Autodesk Inventor part; units mm, degrees
ref_plane "YZ Plane" through (0, 0, 0) normal (1, 0, 0) x (0, 1, 0)
ref_plane "XZ Plane" through (0, 0, 0) normal (0, 1, 0) x (-1, 0, 0)
ref_plane "XY Plane" through (0, 0, 0) normal (0, 0, 1) x (1, 0, 0)
sketch "スケッチ2" plane through (0, 0, 0) normal (1, 0, 0) x (0, 1, 0)
  line L0 (-7.071, 15.2913) -> (-10.3324, 22.2065)
  arc A0 (-10.3324, 22.2065) -> (0.9209, 24.5984) centre (0.1387, 0.6112) ccw
  line L1 (0.9209, 24.5984) -> (0.7542, 16.9546)
  line L2 (0.7542, 16.9546) -> (-7.071, 15.2913)
  circle A1 centre (-8.8613, 0.6112) radius 1.6
  circle A2 centre (9.1387, 0.6112) radius 1.6
  circle A3 centre (0.1387, 0.6112) radius 5.15
  point P0 (0, 0)
extrude "押し出し2" add sketch "スケッチ2" along normal blind 2.5
properties part number "belt_liner_v2_3DP_P-4-F" material "ABS プラスチック"
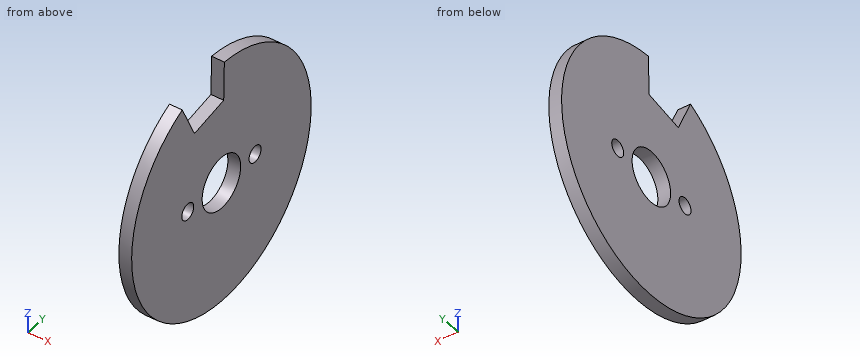
Part model, mm, in its own coordinate system. Round coordinates to 2 decimals unless told otherwise and drop trailing zeros. Write each loop counter-clockwise with the first axis right and the second up, starting at its lowest first coordinate (ties: lowest second). Pieces come first, ordered by that corner, then holes. Notation, with made-up numbers: M 55,87 L 103,87 A16 cw 103,117 Z; hole C 56.5,84 d5. An arc over 180 degrees is marked long. One line per question, with ' | ' between items.
(1) Probe line 1 along Z through (x, y) = (1.75, -3.5); line 2 along Y through (x, z) = (1.85, -4); line 3 along Z through (x, y) = (1.85, 2.5). List the from-to ranges inside material, lowest first.
Answer key:
line 1: z = -23.11 to -3.03, 4.26 to 16.05 | line 2: y = -23.41 to -2.15, 2.43 to 23.69 | line 3: z = -23.27 to -3.97, 5.19 to 24.49
(2) Pin check, flat tips, straight feed: pin 1 (3 mm diameter, centred on y = -7, z = 3.5, fed in from -X); pin 2 (1.5 mm diameter, centred on x = 0.5, z = -1.5, fed in from -Y); pin 3 (1.5 mm diameter, centred on x = 1.5, y = 8.5, fed in from +Z). Stop position of each tip, or through.
Answer key:
pin 1: stops at x = 0 | pin 2: stops at y = -23.82 | pin 3: stops at z = 23.37
(3) Saw through at B-B on z = 3.5. Write the cut outline in (x, y), then the cut area to 3 significant figures.
Answer key:
outline: M 0,-23.69 L 2.5,-23.69 L 2.5,-4.12 L 0,-4.12 Z; M 0,4.4 L 2.5,4.4 L 2.5,23.96 L 0,23.96 Z | area: 97.8 mm^2
(4) Saw through at C-C on x = 1.65. Write the cut outline in (y, z).
Answer key:
outline: M -10.33,22.21 A24 ccw long 0.92,24.6 L 0.75,16.95 L -7.07,15.29 Z; hole C -8.86,0.61 d3.2; hole C 0.14,0.61 d10.3; hole C 9.14,0.61 d3.2
(5) Saw through at D-D on z = -15.5. Write the cut outline in (x, y).
Answer key:
outline: M 0,-17.65 L 2.5,-17.65 L 2.5,17.93 L 0,17.93 Z
(6) Saw through at A-A on y = -0.5. Write the cut outline in (x, z), then the cut area to 3 significant figures.
Answer key:
outline: M 0,-23.38 L 2.5,-23.38 L 2.5,-4.5 L 0,-4.5 Z; M 0,5.72 L 2.5,5.72 L 2.5,16.69 L 0,16.69 Z | area: 74.6 mm^2
